Model file for the job. Use its own axes, mm. Face numbers are marked on the shaded views. A direction names the side the tool comes from. Coordinates: 2 decimals unless noted, no trailing zeros. Write each loop counter-clockwise with the first axis right and the second up, starting at its lowest first coordinate (ties: lowest second). Pieces come first, ordered by that corner, then holes. Notation, with made-up numbers: (37.25, 43.5) - (53.25, 43.5) arc R29 cw to (53.25, 63.5) - close; hole circle Ø5 at (-22.75, -31.5). An arc over 180 degrees is marked (long way). Put each result on its own line as item: value. Start each with the question number.
1. Pull direction X, two halves, no side cores. Call the marked faces 4, 5 and 6: released by +X, released by -X, zero draft, split by the parting line, or undercut.
2. Saw through at C-C, the plane y = 19.5. Write the cut outline in (x, z).
3. Saw through at D-D, the plane y = 25.5. Write the cut outline in (x, z), plus the area to 3 significant figures.
4. Saw through at B-B, the plane z = 2.45. Give the number of separate pieces and of enclosed holes in the cut face, plus the area to 3 significant figures.
5. Drop flat-ended pins along their axis: P1, Ø1, axis at y = 11.5, z = 2.5, coming from the +X side; P2, Ø0.9, axis at x = -29, z = 1.5, coming from the -Y side; P3, Ø1, axis at y = 32, z = 1.5, coming from the -X side; P4, Ø1.5, axis at x = 2, y = 26, coming from the -Z side. Give the stop position or say it passes through.
6. Saw through at A-A, the plane x = 7. Write the cut outline in (y, z), plus the area to 3 significant figures.
7. Which spindle directions (+Z, -Z, +X, -X, +Y, -Y) get a long thin tool onto all of the face, cutting with end or side? Do the marked faces 1, 2 and 3. Say none if no direction does.
8. Drill centre lines: L1, parallel to Y at x = -8.5, z = 2.1; L2, parallel to Y at x = -3, z = 2.4; L3, parallel to Y at x = -31.4, z = 2.05. Where is each one in solid material? Low to high. Write a range as from..to.
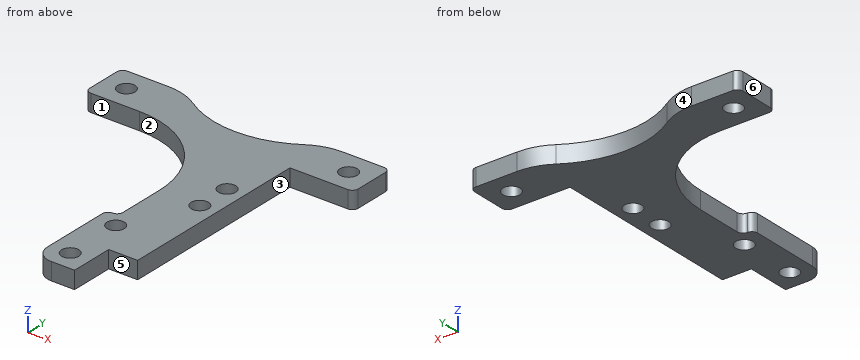
```python
from build123d import *

# Parameters (mm, degrees)
SKETCH_1_R          = 1.5
EXTRUDE_1_DEPTH     = 3
FILLET_1_R          = 1
FILLET_4_R          = 16
SKETCH_2_R          = 17.5
CUT_EXTRUDE_1_DEPTH = 3
FILLET_5_R          = 10
SKETCH_3_W          = 10
SKETCH_3_H          = 7
CUT_EXTRUDE_2_DEPTH = 10
SKETCH_4_W          = 7
SKETCH_4_H          = 1
EXTRUDE_2_DEPTH     = 3
FILLET_7_R          = 3
SKETCH_5_R          = 1.5
CUT_EXTRUDE_3_DEPTH = 10


with BuildPart() as part:
    # 草图1 → 凸台-拉伸1 (new body)
    with BuildSketch(Plane.XY):
        Polygon((0, 0), (0, 3.5), (-5, 3.5), (-5, 13.5), (0, 13.5), (0, 47), (11, 47), (11, 55), (-35.4, 55), (-35.4, 47), (-10, 47), (-10, 22), (-12, 22), (-12, 7), (-10, 7), (-10, 0), align=None)
        with Locations((7, 51)):
            Circle(SKETCH_1_R, mode=Mode.SUBTRACT)
        with Locations((-31.4, 51)):
            Circle(SKETCH_1_R, mode=Mode.SUBTRACT)
        with Locations((-8.5, 19.5)):
            Circle(SKETCH_1_R, mode=Mode.SUBTRACT)
        with Locations((-8.5, 9.5)):
            Circle(SKETCH_1_R, mode=Mode.SUBTRACT)
    extrude(amount=EXTRUDE_1_DEPTH)

    # 圆角1
    fillet_1_edges = [part.edges().sort_by_distance(p)[0] for p in [
        (11, 55, 1.5),
        (11, 47, 1.5),
        (-35.4, 47, 1.5),
        (-35.4, 55, 1.5),
        (-10, 22, 1.5),
        (-12, 22, 1.5),
    ]]
    fillet(fillet_1_edges, radius=FILLET_1_R - 0.0001)  # a hair under: the kernel refuses the full size

    # 圆角4
    fillet_4_edges = [part.edges().sort_by_distance(p)[0] for p in [
        (-10, 47, 1.5),
    ]]
    fillet(fillet_4_edges, radius=FILLET_4_R)

    # 草图2 → 切除-拉伸1 (cut)
    with BuildSketch(Plane.XY.offset(3)):
        with Locations((-12.2, 68)):
            Circle(SKETCH_2_R)
    extrude(amount=-CUT_EXTRUDE_1_DEPTH, mode=Mode.SUBTRACT)

    # 圆角5
    fillet_5_edges = [part.edges().sort_by_distance(p)[0] for p in [
        (-23.915374514, 55, 1.5),
        (-0.484625486, 55, 1.5),
    ]]
    fillet(fillet_5_edges, radius=FILLET_5_R)

    # 草图3 → 切除-拉伸2 (cut)
    with BuildSketch(Plane(origin=(0, 0, 0), x_dir=(-1, 0, 0), z_dir=(0, 0, -1))):
        with Locations((5, 3.5)):
            Rectangle(SKETCH_3_W, SKETCH_3_H)
    extrude(amount=-CUT_EXTRUDE_2_DEPTH, mode=Mode.SUBTRACT)

    # 草图4 → 凸台-拉伸2 (add)
    with BuildSketch(Plane(origin=(0, 0, 0), x_dir=(-1, 0, 0), z_dir=(0, 0, -1))):
        with Locations((8.5, 6.5)):
            Rectangle(SKETCH_4_W, SKETCH_4_H)
    extrude(amount=-EXTRUDE_2_DEPTH)

    # 圆角7
    fillet_7_edges = [part.edges().sort_by_distance(p)[0] for p in [
        (-12, 6, 1.5),
    ]]
    fillet(fillet_7_edges, radius=FILLET_7_R)

    # 草图5 → 切除-拉伸3 (cut)
    with BuildSketch(Plane.XY.offset(3)):
        with Locations((-3, 31)):
            Circle(SKETCH_5_R)
        with Locations((-3, 37)):
            Circle(SKETCH_5_R)
    extrude(amount=-CUT_EXTRUDE_3_DEPTH, mode=Mode.SUBTRACT)


solid = part.part
```
Final values:
1. face 4: undercut
1. face 5: zero draft
1. face 6: released by -X
2. outline: (-12, 0) - (-10, 0) - (-10, 3) - (-12, 3) - close; (-7, 0) - (0, 0) - (0, 3) - (-7, 3) - close
3. outline: (-10, 0) - (0, 0) - (0, 3) - (-10, 3) - close
3. area: 30.0 mm²
4. separate pieces: 1
4. enclosed holes: 6
4. area: 711 mm²
5. P1: stops at x = -5
5. P2: stops at y = 47
5. P3: stops at x = -10.07
5. P4: passes through
6. outline: (47, 0) - (49.5, 0) - (49.5, 3) - (47, 3) - close; (52.5, 0) - (55, 0) - (55, 3) - (52.5, 3) - close
6. area: 15.0 mm²
7. face 1: +Z, -Z, -X, -Y
7. face 2: +Z, -Z, -X
7. face 3: +Z, -Z, +X, -Y
8. L1: y = 6..8, 11..18, 21..50.9
8. L2: y = 13.5..29.5, 32.5..35.5, 38.5..53.11
8. L3: y = 47..49.5, 52.5..55
